Autodesk Inventor part; units mm, degrees
ref_plane "YZ Plane" through (0, 0, 0) normal (1, 0, 0) x (0, 1, 0)
ref_plane "XZ Plane" through (0, 0, 0) normal (0, 1, 0) x (-1, 0, 0)
ref_plane "XY Plane" through (0, 0, 0) normal (0, 0, 1) x (1, 0, 0)
sketch "Sketch9" plane through (0, 0, 0) normal (0, 1, 0) x (-1, 0, 0)
  line L0 (15, 15) -> (-15, 15)
  line L1 (-15, 15) -> (-15, -15)
  line L2 (-15, -15) -> (15, -15)
  line L3 (15, -15) -> (15, 15)
  line L4 (15, 15) -> (-15, -15) construction
  line L5 (-15, 15) -> (15, -15) construction
  line L6 (-13, 13) -> (13, 13)
  line L7 (13, 13) -> (13, -13)
  line L8 (13, -13) -> (-13, -13)
  line L9 (-13, -13) -> (-13, 13)
  point P0 (0, 0)
  dimension "d172" = 30
  dimension "d173" = 30
  dimension "d174" = 2
extrude "Extrusion3" add sketch "Sketch9" against normal blind 270
sketch "Sketch10" plane through (0, 0, 0) normal (1, 0, 0) x (0, 1, 0)
  line L0 (0, 15) -> (0, -15) construction
  line L1 (0, 15) -> (-270, 15) construction
  line L2 (0, -15) -> (-270, -15) construction
  line L3 (-58.5, 8.5) -> (-41.5, 8.5)
  line L4 (-41.5, 8.5) -> (-41.5, -8.5)
  line L5 (-41.5, -8.5) -> (-58.5, -8.5)
  line L6 (-58.5, -8.5) -> (-58.5, 8.5)
  line L7 (-58.5, 8.5) -> (-41.5, -8.5) construction
  line L8 (-41.5, 8.5) -> (-58.5, -8.5) construction
  line L9 (0, 0) -> (30, 0)
  circle A0 centre (-50, 0) radius 8.5
  dimension "d177" = 17
  dimension "d178" = 17
  dimension "d181" = 30
  dimension "d182" = 80
extrude "Extrusion4" cut sketch "Sketch10" along normal through all contours A0
pattern_linear "Rectangular Pattern4" count 4 spacing 68 along (0, -1, 0) of "Extrusion4"
properties part number "PRS 1200-56 FDS 1000 way tube 4" material "Stainless Steel"
Geometry check sheet. Reference: the model listing, model coordinates, mm. A direction names the side the tool comes from. Give positions to 0.01 mm unless a question says otherwise; leave off trailing zeros. Write each loop counter-clockwise with the first axis right and the second up, starting at its lowest first coordinate (ties: lowest second). Pieces come first, ordered by that corner, then holes. Notation, with made-up numbers: (23.5, 85.5) - (45.5, 85.5) arc R5 cw to (45.5, 90.5) - close; hole circle Ø7 at (-28, 59.5). An arc over 180 degrees is marked (long way). Put each result on its own line as item: value.
1. Sectioned sample at B-B, the plane z = 5.5. Enter the section's corners in (x, y).
Ans:
outline: (-15, -270) - (-13, -270) - (-13, 0) - (-15, 0) - close; (13, -270) - (15, -270) - (15, -260.48) - (13, -260.48) - close; (13, -247.52) - (15, -247.52) - (15, -192.48) - (13, -192.48) - close; (13, -179.52) - (15, -179.52) - (15, -124.48) - (13, -124.48) - close; (13, -111.52) - (15, -111.52) - (15, -56.48) - (13, -56.48) - close; (13, -43.52) - (15, -43.52) - (15, 0) - (13, 0) - close
2. Draft check along Z on faces 1 (the flat face through (15, -133, 0)), 2 (the flat face through (0, -133, -15)), 3 (the flat face through (0, -133, 13)). Enter one of: +Z half, -Z half, draft (parallel to the pull), parting line (faces both ways), or undercut.
Ans:
face 1: draft
face 2: -Z half
face 3: undercut
3. Sectioned sample at C-C, the plane y = -174.5. Enter the section's corners in (x, z), plus the area to 3 significant figures.
Ans:
outline: (-15, -15) - (15, -15) - (15, 15) - (-15, 15) - close; hole (-13, -13) - (13, -13) - (13, 13) - (-13, 13) - close
area: 224 mm²
4. Set-up check for faces 4 (the flat face through (0, -133, -13)), 5 (the flat face through (14, -270, 0)), 6 (the cylindrical face through (13.99, -262.49, -0.37)): record each of +Z, -Z, +X, -X, +Y, -Y from which the full face is reachable in a straight line by a thin tool's end or side.
Ans:
face 4: +Y, -Y
face 5: +Z, -Z, +X, -X, -Y
face 6: +X
5. Sectioned sample at A-A, the plane x = 4.5. Enter the section's corners in (y, z), plus the area to 3 significant figures.
Ans:
outline: (-270, -15) - (0, -15) - (0, -13) - (-270, -13) - close; (-270, 13) - (0, 13) - (0, 15) - (-270, 15) - close
area: 1,080 mm²
6. Thickness scan on line 1 (Y direction, x = 14.6, z = 0); line 2 (X direction, y = -97, z = 11.75); line 3 (Z direction, x = 13.9, y = -186). Record the ranges inside material, lowest first.
Ans:
line 1: y = -270 to -262.5, -245.5 to -194.5, -177.5 to -126.5, -109.5 to -58.5, -41.5 to 0
line 2: x = -15 to -13, 13 to 15
line 3: z = -15 to -8.5, 8.5 to 15
7. Go/stop test with a flat-tipped pin: pin 1 (13.5 mm diameter, centred on y = -118, z = 0, fed in from +X). Record where the tip stops, or that it passes through.
Ans:
pin 1: stops at x = -13
8. Sectioned sample at D-D, the plane y = -50. Enter the section's corners in (x, z).
Ans:
outline: (-15, -15) - (15, -15) - (15, -8.5) - (13, -8.5) - (13, -13) - (-13, -13) - (-13, 13) - (13, 13) - (13, 8.5) - (15, 8.5) - (15, 15) - (-15, 15) - close
